CAD build for the part. Positions are in the model's coordinates, mm. A direction names the side the tool comes from. Round coordinates to 2 decimals unless told otherwise and drop trailing zeros. Write each loop counter-clockwise with the first axis right and the second up, starting at its lowest first coordinate (ties: lowest second). Pieces come first, ordered by that corner, then holes. Notation, with made-up numbers: (76, 42.25) - (115, 42.25) arc R21 cw to (115, 73.25) - close; hole circle Ø8 at (59.5, -13.5). An arc over 180 degrees is marked (long way). Answer in a Markdown table with one row per item.
```python
from build123d import *

# Parameters (mm, degrees)
SKETCH1_W           = 46
SKETCH1_H           = 32
SKETCH1_R           = 1.6
SKETCH1_R_2         = 8
EXTRUDE1_DEPTH      = 5
SKETCH2_W           = 10
SKETCH2_H           = 8
EXTRUDE2_DEPTH      = 29.460498942
EXTRUDE3_DEPTH      = 23
SKETCH4_R           = 1.6
EXTRUDE4_DEPTH      = 48.741491389
SKETCH_1_W          = 12.5
SKETCH_1_H          = 58
SKETCH_1_R          = 1.6
EXTRUDE_1_DEPTH     = 4
CUT_EXTRUDE_1_DEPTH = 10
FILLET_1_R          = 2


with BuildPart() as part:
    # Sketch1 → Extrude1 (new body)
    with BuildSketch(Plane(origin=(0, 0, 0), x_dir=(0, 0, -1), z_dir=(1, 0, 0))):
        Rectangle(SKETCH1_W, SKETCH1_H)
        with Locations((16, 9.5)):
            Circle(SKETCH1_R, mode=Mode.SUBTRACT)
        with Locations((-17, 9.5)):
            Circle(SKETCH1_R, mode=Mode.SUBTRACT)
        with Locations((-8, 0.5)):
            Circle(SKETCH1_R_2, mode=Mode.SUBTRACT)
        with Locations(Location((-17, -8.5, 0), (0, 0, 180))):
            Circle(SKETCH1_R, mode=Mode.SUBTRACT)
        with Locations(Location((16, -8.5, 0), (0, 0, 180))):
            Circle(SKETCH1_R, mode=Mode.SUBTRACT)
    extrude(amount=EXTRUDE1_DEPTH)

    # Sketch2 → Extrude2 (cut, through all)
    with BuildSketch(Plane(origin=(5, 0, 0), x_dir=(0, 0, -1), z_dir=(1, 0, 0))):
        with Locations((-18, 0.5)):
            Rectangle(SKETCH2_W, SKETCH2_H)
    extrude(amount=-EXTRUDE2_DEPTH, mode=Mode.SUBTRACT)

    # Sketch3 → Extrude3 (add, symmetric)
    with BuildSketch(Plane.XY):
        Polygon((0, -16), (0, -22), (-12.5, -22), (-12.5, -26), (17.5, -26), (17.5, -22), (5, -22), (5, -16), align=None)
    extrude(amount=EXTRUDE3_DEPTH, both=True)

    # Sketch4 → Extrude4 (cut, through all)
    with BuildSketch(Plane(origin=(0, -22, 0), x_dir=(1, 0, 0), z_dir=(0, 1, 0))):
        with Locations(Location((-7.5, -12.5, 0), (0, 0, 270))):
            Circle(SKETCH4_R)
        with Locations(Location((12.5, -12.5, 0), (0, 0, 90))):
            Circle(SKETCH4_R)
        with Locations(Location((-7.5, 12.5, 0), (0, 0, 90))):
            Circle(SKETCH4_R)
        with Locations(Location((12.5, 12.5, 0), (0, 0, 270))):
            Circle(SKETCH4_R)
    extrude(amount=-EXTRUDE4_DEPTH, mode=Mode.SUBTRACT)

    # 草图1 → 凸台-拉伸1 (add)
    with BuildSketch(Plane.XZ.offset(26)):
        with Locations((-6.25, 0)):
            Rectangle(SKETCH_1_W, SKETCH_1_H)
        with Locations((-7.5, -25)):
            Circle(SKETCH_1_R, mode=Mode.SUBTRACT)
        with Locations(Location((-7.5, 25, 0), (0, 0, 270))):
            Circle(SKETCH_1_R, mode=Mode.SUBTRACT)
    extrude(amount=-EXTRUDE_1_DEPTH)

    # 草图2 → 切除-拉伸1 (cut)
    with BuildSketch(Plane(origin=(0, -22, 0), x_dir=(1, 0, 0), z_dir=(0, 1, 0))):
        with BuildLine():
            Line((-12.5, 16), (-12.5, -16))
            ThreePointArc((-12.5, -16), (-4.5, 0), (-12.5, 16))
        make_face()
    extrude(amount=-CUT_EXTRUDE_1_DEPTH, mode=Mode.SUBTRACT)

    # 圆角1
    fillet_1_edges = [part.edges().sort_by_distance(p)[0] for p in [
        (0, -24, 29),
        (-12.5, -24, -29),
        (0, -24, -29),
        (0, -24, -23),
        (0, -24, 23),
        (-12.5, -24, 29),
        (17.5, -24, -23),
        (17.5, -24, 23),
        (2.5, 16, 23),
        (2.5, 16, -23),
    ]]
    fillet(fillet_1_edges, radius=FILLET_1_R)


solid = part.part
```
Q1. Pull direction Y, two halves, no side cores. Call faces 6 (the flat face through (2, 9, 23)), 7 (the flat face through (-4, -22, 0)), 8 (the cylindrical face through (2.465, 0.207, 0.005)): released by +Y, released by -Y, zero draft, split by the parting line, or undercut.
Computed:
| item | result |
|---|---|
| face 6 | zero draft |
| face 7 | released by +Y |
| face 8 | undercut |
Q2. Saw through at C-C on z = 12.5. List the corners of the cut face in (x, y), then the cut area to 3 significant figures.
Computed:
| item | result |
|---|---|
| outline | (-8.89, -26) - (10.9, -26) - (10.9, -22) - (5, -22) - (5, -6.11) - (0, -6.11) - (0, -22) - (-8.89, -22) - close; (0, 7.11) - (5, 7.11) - (5, 16) - (0, 16) - close; (14.1, -26) - (17.5, -26) - (17.5, -22) - (14.1, -22) - close |
| area | 217 mm2 |
Q3. Saw through at B-B on x = -7.5. List the corners of the cut face in (y, z).
Computed:
| item | result |
|---|---|
| outline | (-26, -29) - (-22, -29) - (-22, -26.6) - (-26, -26.6) - close; (-26, -23.4) - (-22, -23.4) - (-22, -10.54) - (-26, -10.54) - close; (-26, 10.54) - (-22, 10.54) - (-22, 23.4) - (-26, 23.4) - close; (-26, 26.6) - (-22, 26.6) - (-22, 29) - (-26, 29) - close |
Q4. Saw through at A-A on y = 9.5. List the corners of the cut face in (x, z), then the cut area to 3 significant figures.
Computed:
| item | result |
|---|---|
| outline | (0, -23) - (5, -23) - (5, -17.6) - (0, -17.6) - close; (0, -14.4) - (5, -14.4) - (5, 15.4) - (0, 15.4) - close; (0, 18.6) - (5, 18.6) - (5, 23) - (0, 23) - close |
| area | 198 mm2 |
Q5. Saw through at D-D on z = -4. List the corners of the cut face in (x, y).
Computed:
| item | result |
|---|---|
| outline | (-4.9, -26) - (17.5, -26) - (17.5, -22) - (5, -22) - (5, 16) - (0, 16) - (0, -22) - (-4.9, -22) - close |
Q6. Drill centre lines: line 1 (Y direction, x = 3.55, z = 17); line 2 (Y direction, x = 2.8, z = -16); line 3 (Y direction, x = 2.3, z = 8). Where is each one in solid material? Low to high.
Computed:
| item | result |
|---|---|
| line 1 | y = -26 to -10.1, -6.9 to -3.5, 4.5 to 7.9, 11.1 to 16 |
| line 2 | y = -26 to -10.1, -6.9 to 7.9, 11.1 to 16 |
| line 3 | y = -26 to -7.5, 8.5 to 16 |
Q7. 3-axis set-ups, long thin cutter, end or side, ignore diameter. For faces 1 (the cylindrical face through (12.43, -23.97, 14.1)), 2 (the flat face through (4, -17, 23)), 3 (the flat face through (3, -3.5, 19)), 4 (the cylindrical face through (-0.6, -23.97, 28.43)), 5 (the flat face through (0, -24, -26)): which of +Z, -Z, +X, -X, +Y, -Y reach the whole face in a straight line?
Computed:
| item | result |
|---|---|
| face 1 | +Y, -Y |
| face 2 | +Z, +X, +Y |
| face 3 | +Z, +X, -X |
| face 4 | +Z, +X, +Y, -Y |
| face 5 | -Z, +X, +Y, -Y |
Q8. Flat gauge pins, fed straight in: pin 1 (3.5 mm diameter, centred on x = 12.5, z = -12.5, fed in from -Y); pin 2 (10 mm diameter, centred on x = -6, z = -11, fed in from +Y); pin 3 (3 mm diameter, centred on x = -1, y = -15, fed in from -Z); pin 4 (4 mm diameter, centred on y = 5.5, z = -9, fed in from -X). Where does each tip first touch, or does it go through?
Computed:
| item | result |
|---|---|
| pin 1 | stops at y = -26 |
| pin 2 | stops at y = -22 |
| pin 3 | stops at z = -23 |
| pin 4 | stops at x = 0 |
